CAD build for the part. Positions are in the model's coordinates, mm. A direction names the side the tool comes from. Coordinates: 2 decimals unless noted, no trailing zeros. Loops run counter-clockwise (first coordinate to the right, second up) from the corner with the lowest first, then second, coordinate; pieces in that order, holes last. Notation, with made-up numbers: (-9.75, -33.5) -> (29.25, -33.5) arc R22 ccw to (29.25, -24.5) -> close; hole circle Ø9 at (70, 7). An arc over 180 degrees is marked (long way). Return JSON: item names as keys, results as strings. Group by question number.
(1) Saw through at D-D on x = -33.5. Write the cut outline in (y, z), then the cut area to 3 significant figures.
(2) Saw through at A-A on y = 14.5. Write the cut outline in (x, z).
(3) Tool access for faces 4 (the face through (-91, 5, -1)), 5 (the face through (113, 54, -2)): list every direction of +Z, -Z, +X, -X, +Y, -Y with a clear straight run to the whole face (end or side of a thin tool).
(4) Mould opens along X. For faces 1 (the face through (-2, 1, 0)), 2 (the face through (-114, 53, -2)), 3 (the face through (-105.854, -47.324, -1.479)) say: pulls with the +X half, pulls with the -X half, needs draft (parallel to the pull), parting line crosses it, or undercut.
(5) Saw through at B-B on x = 91. Write the cut outline in (y, z), then the cut area to 3 significant figures.
(6) Saw through at C-C on z = -1.8. Give the number of separate pieces and of enclosed holes in the cut face, then the cut area to 3 significant figures.
(7) Probe L1, parallel to Y at x = -108, z = -2; L2, parallel to X at y = 24.5, z = -2.6; L3, parallel to Y at x = 91, z = -1.4. List the from-to ranges inside material, lowest first.
(8) Flat gauge pin, fed straight in: pin 1 Ø3.5 at (x, y) = (-108, -48) entering from -Z. Where does the tip first touch, or does it go through?
Autodesk Inventor part; units mm, degrees
ref_plane "YZ Plane" through (0, 0, 0) normal (1, 0, 0) x (0, 1, 0)
ref_plane "XZ Plane" through (0, 0, 0) normal (0, 1, 0) x (-1, 0, 0)
ref_plane "XY Plane" through (0, 0, 0) normal (0, 0, 1) x (1, 0, 0)
sketch "Sketch1" plane through (0, 0, 0) normal (0, 0, 1) x (1, 0, 0)
  line L0 (-92.5, -50) -> (92.5, -50)
  line L1 (92.5, -50) -> (92.5, 50)
  line L2 (92.5, 50) -> (-92.5, 50)
  line L3 (-92.5, 50) -> (-92.5, -50)
  line L4 (-92.5, -50) -> (92.5, 50) construction
  line L5 (92.5, -50) -> (-92.5, 50) construction
  line L6 (70, 55) -> (115, 55)
  line L7 (115, 55) -> (115, 45)
  line L8 (115, 45) -> (70, 45)
  line L9 (70, 45) -> (70, 55)
  line L10 (70, 55) -> (115, 45) construction
  line L11 (115, 55) -> (70, 45) construction
  line L12 (70, -45) -> (115, -45)
  line L13 (115, -45) -> (115, -55)
  line L14 (115, -55) -> (70, -55)
  line L15 (70, -55) -> (70, -45)
  line L16 (70, -45) -> (115, -55) construction
  line L17 (115, -45) -> (70, -55) construction
  line L18 (-115, -45) -> (-70, -45)
  line L19 (-70, -45) -> (-70, -55)
  line L20 (-70, -55) -> (-115, -55)
  line L21 (-115, -55) -> (-115, -45)
  line L22 (-115, -45) -> (-70, -55) construction
  line L23 (-70, -45) -> (-115, -55) construction
  line L24 (-115, 55) -> (-70, 55)
  line L25 (-70, 55) -> (-70, 45)
  line L26 (-70, 45) -> (-115, 45)
  line L27 (-115, 45) -> (-115, 55)
  line L28 (-115, 55) -> (-70, 45) construction
  line L29 (-70, 55) -> (-115, 45) construction
  line L30 (70, 45) -> (115, 45)
  line L31 (115, 45) -> (115, -45)
  line L32 (115, -45) -> (70, -45)
  line L33 (70, -45) -> (70, 45)
  line L34 (70, 45) -> (115, -45) construction
  line L35 (115, 45) -> (70, -45) construction
  line L36 (-115, 45) -> (-70, 45)
  line L37 (-70, 45) -> (-70, -45)
  line L38 (-70, -45) -> (-115, -45)
  line L39 (-115, -45) -> (-115, 45)
  line L40 (-115, 45) -> (-70, -45) construction
  line L41 (-70, 45) -> (-115, -45) construction
  line L42 (115, 45) -> (115, 25)
  line L43 (115, -45) -> (115, -25)
  line L44 (-115, -45) -> (-115, -25)
  line L45 (-115, 45) -> (-115, 25)
  line L46 (70, 55) -> (-70, 55)
  line L47 (-70, 55) -> (-70, 50)
  line L48 (-70, 50) -> (70, 50)
  line L49 (70, 50) -> (70, 55)
  point P0 (0, 0)
  point P1 (0, 0)
  point P2 (92.5, 0)
  point P3 (-92.5, 0)
  point P4 (-70, -50)
  point P5 (70, -50)
  dimension "d0" = 185
  dimension "d1" = 100
  dimension "d2" = 45
  dimension "d3" = 10
  dimension "d4" = 45
  dimension "d5" = 10
  dimension "d6" = 45
  dimension "d7" = 45
  dimension "d8" = 10
  dimension "d9" = 45
  dimension "d10" = 90
  dimension "d11" = 20
  dimension "d12" = 20
  dimension "d13" = 20
  dimension "d14" = 20
  dimension "d15" = 45
extrude "Extrusion1" add sketch "Sketch1" against normal blind 3
fillet "Fillet1" radius 5 8 edges at (-115, 55, -1.5) (115, 55, -1.5) (115, -55, -1.5) (70, -55, -1.5) (70, -50, -1.5) (-70, -50, -1.5) (-70, -55, -1.5) (-115, -55, -1.5)
sketch "Sketch2" plane through (0, 0, 0) normal (0, 0, 1) x (1, 0, 0)
  circle A0 centre (-91, 40) radius 5
  circle A1 centre (-91, 10) radius 5
  line L0 (-96, 40) -> (-96, 10)
  line L1 (-86, 10) -> (-86, 40)
  line L2 (-73.6603, 55) -> (-110, 55)
  line L3 (-115, 50) -> (-115, -50)
  circle A2 centre (-108, 48) radius 2.25
  line L4 (0, 60.4736) -> (0, -65.7733) construction
  circle A3 centre (91, 40) radius 5
  circle A4 centre (91, 10) radius 5
  line L5 (96, 40) -> (96, 10)
  line L6 (86, 10) -> (86, 40)
  circle A5 centre (108, 48) radius 2.25
  line L7 (-147.6516, 0) -> (131.888, 0) construction
  circle A6 centre (-108, -48) radius 2.25
  circle A7 centre (108, -48) radius 2.25
  point P0 (0, 0)
  dimension "d19" = 10
  dimension "d20" = 10
  dimension "d24" = 15
  dimension "d25" = 24
  dimension "d26" = 24
  dimension "d27" = 19
  dimension "d28" = 45
  dimension "d32" = 7
  dimension "d33" = 7
extrude "Extrusion2" cut sketch "Sketch2" against normal blind 3
properties part number "CONTROLBOARD_KLEP"
Geometry results:
{
 "1": {"outline": "(-50, -3) -> (55, -3) -> (55, 0) -> (-50, 0) -> close", "area": "315 mm²"},
 "2": {"outline": "(-115, -3) -> (-96, -3) -> (-96, 0) -> (-115, 0) -> close; (-86, -3) -> (86, -3) -> (86, 0) -> (-86, 0) -> close; (96, -3) -> (115, -3) -> (115, 0) -> (96, 0) -> close"},
 "3": {"face 4": "+Z, -Z", "face 5": "+Z, -Z, +X, +Y"},
 "4": {"face 1": "needs draft", "face 2": "pulls with the -X half", "face 3": "undercut"},
 "5": {"outline": "(-55, -3) -> (5, -3) -> (5, 0) -> (-55, 0) -> close; (45, -3) -> (55, -3) -> (55, 0) -> (45, 0) -> close", "area": "210 mm²"},
 "6": {"separate pieces": "1", "enclosed holes": "6", "area": "23,800 mm²"},
 "7": {"L1": "-55 to -50.25, -45.75 to 45.75, 50.25 to 55", "L2": "-115 to -96, -86 to 86, 96 to 115", "L3": "-55 to 5, 45 to 55"},
 "8": {"pin 1": "through"}
}
